```python
from build123d import *

# Parameters (mm, degrees)
SKETCH1_R           = 27
SKETCH1_R_2         = 25.4
EXTRUDE_THIN1_DEPTH = 120
BOSS_EXTRUDE1_START = -2
BOSS_EXTRUDE1_DEPTH = 2
BOSS_EXTRUDE2_DEPTH = 2
SKETCH4_R           = 12.5
CUT_EXTRUDE2_DEPTH  = 31
SKETCH5_R           = 5
CUT_EXTRUDE3_DEPTH  = 18
SKETCH6_R           = 5
CUT_EXTRUDE4_DEPTH  = 18


with BuildPart() as part:
    # Sketch1 → Extrude-Thin1 (new body)
    with BuildSketch(Plane.XY):
        Circle(SKETCH1_R)
        Circle(SKETCH1_R_2, mode=Mode.SUBTRACT)
    extrude(amount=EXTRUDE_THIN1_DEPTH)

    # Sketch2 → Boss-Extrude1 (add)
    with BuildSketch(Plane.XY.offset(120).offset(BOSS_EXTRUDE1_START)):
        with BuildLine():
            Line((21.964447337, 12.756294649), (-21.964447337, 12.756294649))
            ThreePointArc((-21.964447337, 12.756294649), (-6.60541587, -24.526077574), (25.4, 0))
            ThreePointArc((25.4, 0), (24.526077574, 6.60541587), (21.964447337, 12.756294649))
        make_face()
    extrude(amount=BOSS_EXTRUDE1_DEPTH)

    # Sketch3 → Boss-Extrude2 (add)
    with BuildSketch(Plane(origin=(0, 0, 0), x_dir=(-1, 0, 0), z_dir=(0, 0, -1))):
        with BuildLine():
            ThreePointArc((25.4, 0), (24.526077574, 6.60541587), (21.964447337, 12.756294649))
            Line((21.964447337, 12.756294649), (-21.964447337, 12.756294649))
            ThreePointArc((-21.964447337, 12.756294649), (-6.60541587, -24.526077574), (25.4, 0))
        make_face()
    extrude(amount=-BOSS_EXTRUDE2_DEPTH)

    # Sketch4 → Cut-Extrude2 (cut)
    with BuildSketch(Plane(origin=(0, 0, 0), x_dir=(1, 0, 0), z_dir=(0, 1, 0))):
        with Locations(Location((0, -14.899672821, 0), (0, 0, 90))):
            Circle(SKETCH4_R)
        with Locations(Location((0, -44.899672821, 0), (0, 0, 90))):
            Circle(SKETCH4_R)
        with Locations(Location((0, -74.899672821, 0), (0, 0, 90))):
            Circle(SKETCH4_R)
        with Locations(Location((0, -104.899672821, 0), (0, 0, 90))):
            Circle(SKETCH4_R)
    extrude(amount=CUT_EXTRUDE2_DEPTH, mode=Mode.SUBTRACT)

    # Sketch5 → Cut-Extrude3 (cut)
    with BuildSketch(Plane(origin=(0, 0, 0), x_dir=(-1, 0, 0), z_dir=(0, 0, -1))):
        with Locations((0, 5)):
            Circle(SKETCH5_R)
    extrude(amount=-CUT_EXTRUDE3_DEPTH, mode=Mode.SUBTRACT)

    # Sketch6 → Cut-Extrude4 (cut)
    with BuildSketch(Plane.XY.offset(120)):
        with Locations((0, -5)):
            Circle(SKETCH6_R)
    extrude(amount=-CUT_EXTRUDE4_DEPTH, mode=Mode.SUBTRACT)


solid = part.part
```
Can you work these out from the model? Positions are in its coordinate system, mm. A direction names the side the tool comes from. Coordinates: 2 decimals unless noted, no trailing zeros. Loops run counter-clockwise (first coordinate to the right, second up) from the corner with the lowest first, then second, coordinate; pieces in that order, holes last. Notation, with made-up numbers: (33, -1.75) - (51, -1.75) arc R15 ccw to (51, 15.25) - close; hole circle Ø4 at (20, 87). An arc over 180 degrees is marked (long way). Use a Markdown table: item, result.
Item 1: For faces 5 (the face through (11.721, -22.534, 59.16)), 6 (the face through (7.606, 24.521, 84.819)), 7 (the face through (-4, -8, 119)), which set-ups out of +Z, -Z, +X, -X, +Y, -Y let a thin tool reach every point of the face, with its end or its side?
Numbers:
| item | result |
|---|---|
| face 5 | none |
| face 6 | +Y |
| face 7 | +Z |
Item 2: I want a section at D-D on z = 18. Please give me the cut outline in (x, y), and give its area (3 significant figures).
Numbers:
| item | result |
|---|---|
| outline | (-12.11, 22.33) - (-12.11, 24.13) arc R27 ccw (long way) to (12.11, 24.13) - (12.11, 22.33) arc R25.4 cw (long way) to start |
| area | 223 mm2 |
Item 3: Will these pins go through, and if not, where does the flat tip stop? pin 1 (0.6 mm diameter, centred on x = -3.5, z = 119, fed in from +Y); pin 2 (8 mm diameter, centred on y = -21, z = 69.5, fed in from +X); pin 3 (15 mm diameter, centred on x = 0, z = 104.9, fed in from +Y).
Numbers:
| item | result |
|---|---|
| pin 1 | stops at y = 26.81 |
| pin 2 | stops at x = 20.98 |
| pin 3 | stops at y = -24.27 |
Item 4: We'd pull the mould along X, two halves only. Please class faces 1 (the face through (-5.85, -26.36, 59.16)), 2 (the face through (1.08, 0.12, 0.99)), 3 (the face through (-0.4, 0.4, 120)), 4 (the face through (0, -6, 2)): released by +X, released by -X, zero draft, split by the parting line, or undercut.
Numbers:
| item | result |
|---|---|
| face 1 | split by the parting line |
| face 2 | undercut |
| face 3 | zero draft |
| face 4 | undercut |
Item 5: I want a section at A-A on y = 17.5. Please give me the cut outline in (x, z), and give its area (3 significant figures).
Numbers:
| item | result |
|---|---|
| outline | (-20.56, 0) - (-18.41, 0) - (-18.41, 120) - (-20.56, 120) - close; (18.41, 0) - (20.56, 0) - (20.56, 120) - (18.41, 120) - close |
| area | 516 mm2 |
Item 6: I want a section at C-C on y = -5. Please give me the cut outline in (x, z).
Numbers:
| item | result |
|---|---|
| outline | (-26.53, 0) - (26.53, 0) - (26.53, 120) - (5, 120) - (5, 118) - (24.9, 118) - (24.9, 2) - (-24.9, 2) - (-24.9, 118) - (-5, 118) - (-5, 120) - (-26.53, 120) - close |
Item 7: If I drill on probe 1 along Z at (x, y) = (-5.5, -4); probe 2 along Y at (x, z) = (0, 119.2); probe 3 along X at (y, z) = (-0.5, 12), over which ranges is the centre line in solid material (lowest first)? Write a range as from..to.
Numbers:
| item | result |
|---|---|
| probe 1 | z = 0..2, 118..120 |
| probe 2 | y = -27..-10, 0..12.76, 25.4..27 |
| probe 3 | x = -27..-25.4, 25.4..27 |
Item 8: I want a section at B-B on x = -19. Please give me the cut outline in (y, z).
Numbers:
| item | result |
|---|---|
| outline | (-19.18, 0) - (12.76, 0) - (12.76, 2) - (-16.86, 2) - (-16.86, 118) - (12.76, 118) - (12.76, 120) - (-19.18, 120) - close; (16.86, 0) - (19.18, 0) - (19.18, 120) - (16.86, 120) - close |
